For this review, take the finished solid that the model builds, in its own axes (mm). A direction names the side the tool comes from. Coordinates: 2 decimals unless noted, no trailing zeros. Loops run counter-clockwise (first coordinate to the right, second up) from the corner with the lowest first, then second, coordinate; pieces in that order, holes last. Notation, with made-up numbers: M 83.25,46.25 L 136.25,46.25 A23 cw 136.25,64.25 Z; hole C 52,69 d10. An arc over 180 degrees is marked long. Write each question's results on one line, items separated by ' | '. Start each with the question number.
Autodesk Inventor part; units mm, degrees
ref_plane "YZ Plane" through (0, 0, 0) normal (1, 0, 0) x (0, 1, 0)
ref_plane "XZ Plane" through (0, 0, 0) normal (0, 1, 0) x (-1, 0, 0)
ref_plane "XY Plane" through (0, 0, 0) normal (0, 0, 1) x (1, 0, 0)
sketch "Sketch1" plane through (0, 0, 0) normal (0, 0, 1) x (1, 0, 0)
  line L0 (-206.4033, 0) -> (746.0967, 0)
  line L1 (746.0967, 0) -> (746.0967, 117.475)
  line L2 (746.0967, 117.475) -> (-206.4033, 117.475)
  line L3 (-206.4033, 117.475) -> (-206.4033, 0)
  point P0 (0, 0)
  dimension "d0" = 952.5
  dimension "d1" = 117.475
extrude "Extrusion1" add sketch "Sketch1" along normal blind 95.25
sketch "Sketch3" plane through (-206.4033, 117.475, 0) normal (0, 1, 0) x (1, 0, 0)
  line L0 (952.5, 0) -> (0, 0)
  line L1 (0, 0) -> (95.25, 0)
  line L2 (952.5, -95.25) -> (0, -95.25)
  line L3 (95.25, 0) -> (0, -95.25)
  line L4 (952.5, 0) -> (857.25, 0)
  line L5 (857.25, 0) -> (952.5, -95.25)
  line L6 (0, -95.25) -> (0, 0)
  line L7 (0, 0) -> (95.25, 0)
  line L8 (857.25, 0) -> (952.5, 0)
  line L9 (952.5, 0) -> (952.5, -95.25)
  line L10 (95.25, 0) -> (857.25, 0)
  point P0 (206.4033, 0)
  dimension "d6" = 95.25
  dimension "d7" = 95.25
extrude "Extrusion2" cut sketch "Sketch3" against normal through all contours L9 L5 L0 | L3 L6 L0
fillet "Fillet1" radius 34.925 2 edges at (269.8467, 0, 95.25) (269.8467, 117.475, 95.25)
shell "Shell1" [suppressed]
sketch "Sketch4" plane through (-111.1533, 117.475, 0) normal (0, 1, 0) x (1, 0, 0)
  line L0 (762, 0) -> (0, 0)
  line L1 (381, 0) -> (381, 381)
  point P0 (111.1533, 0)
ref_plane "Work Plane1" through (269.8467, 107.475, -381) normal (0, 0, -1) x (0, 1, 0)
pattern_circular "Circular Pattern1" count 4 over 360 about axis through (269.8467, 107.475, -381) along (0, 1, 0)
fillet "Fillet3" radius 34.925 12 edges at (-196.174, 107.2457, -847.0207) (-196.174, 10.2293, -847.0207) (-206.4033, 58.7375, -857.25) (746.0967, 58.7375, -857.25) (735.8674, 10.2293, -847.0207) (735.8674, 107.2457, -847.0207) (735.8674, 107.2457, 85.0207) (735.8674, 10.2293, 85.0207) (746.0967, 58.7375, 95.25) (-196.174, 10.2293, 85.0207) (-196.174, 107.2457, 85.0207) (-206.4033, 58.7375, 95.25)
properties part number "2025 Bumper Fabric"
Q1. Take a section at A-A, the plane x = 129.5. Give the boundary of the cut face in (y, z) (3 decimals), then the cut area to 3 significant figures.
Q2. To check wall thickness, follow line 1 along Z through (x, y) = (198.5, 64.5); line 2 along X through (y, z) = (57, -240); line 3 along X through (y, z) = (92.5, -347). State the ranges of each line that lie inside material, in increasing order.
Q3. Take a section at B-B, the plane y = 54. Give the boundary of the cut face in (x, z) (3 decimals).
Q4. For faces 1 (the face through (276.025, 106.973, -847.291)), 2 (the face through (275, 60, -762)), list the 3-axis set-ups (+Z, -Z, +X, -X, +Y, -Y) from which the entire face can be reached by the end or side of a thin tool; tool diameter is ignored.
Q5. The part is to be moulded in two halves that separate along Z. For faces 3 (the face through (736.137, 10.502, -387.179)), 4 (the face through (735.594, 58.404, -847.291)), 5 (the face through (-111.153, 60, -386)), 6 (the face through (276.03, 10.5, 85.29)), say which applies: pulls with the +Z half, pulls with the -Z half, needs draft (parallel to the pull), parting line crosses it, or undercut.
Q6. Take a section at C-C, the plane z = -696. Give the boundary of the cut face in (x, y) (3 decimals), then the cut area to 3 significant figures.
Results:
1) outline: M 0,-822.325 A34.925 ccw 34.925,-857.25 L 82.55,-857.25 A34.925 ccw 117.475,-822.325 L 117.475,-762 L 0,-762 Z; M 0,0 L 117.475,0 L 117.475,60.325 A34.925 ccw 82.55,95.25 L 34.925,95.25 A34.925 ccw 0,60.325 Z | area: 21,300 mm^2
2) line 1: -857.25 to -762, 0 to 95.25 | line 2: -206.4 to -111.15, 650.85 to 746.1 | line 3: -204.96 to -111.15, 650.85 to 744.65
3) outline: M -206.403,-822.325 A34.925 ccw -171.478,-857.25 L 711.172,-857.25 A34.925 ccw 746.097,-822.325 L 746.097,60.325 A34.925 ccw 711.172,95.25 L -171.478,95.25 A34.925 ccw -206.403,60.325 Z; hole M -111.153,-762 L 650.847,-762 L 650.847,0 L -111.153,0 Z
4) face 1: -Z, +X, -X, +Y | face 2: +Y, -Y
5) face 3: needs draft | face 4: pulls with the -Z half | face 5: undercut | face 6: pulls with the +Z half
6) outline: M -206.403,34.925 A34.925 ccw -171.478,0 L -111.153,0 L -111.153,117.475 L -171.478,117.475 A34.925 ccw -206.403,82.55 Z; M 650.847,0 L 711.172,0 A34.925 ccw 746.097,34.925 L 746.097,82.55 A34.925 ccw 711.172,117.475 L 650.847,117.475 Z | area: 21,300 mm^2
